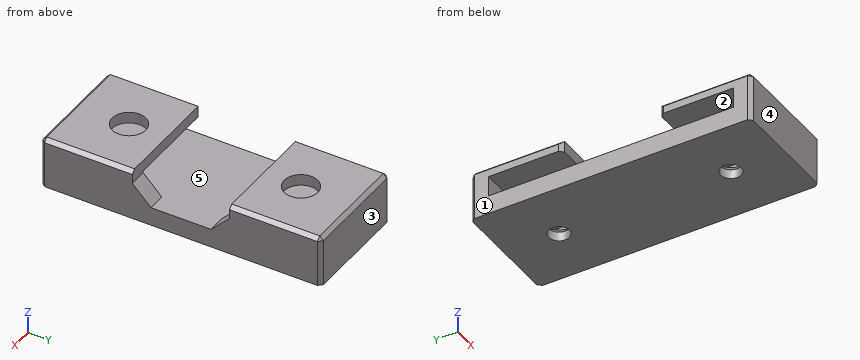
from build123d import *

# Parameters (mm, degrees)
SKETCH001_W     = 30
SKETCH001_H     = 75
SKETCH001_R     = 2.75
PAD_DEPTH       = 5
PAD001_DEPTH    = 5.5
SKETCH003_W     = 30
SKETCH003_H     = 24.5
PAD002_DEPTH    = 3
CHAMFER_SIZE    = 2.5
SKETCH004_R     = 4.5
POCKET_DEPTH    = 3
CHAMFER001_SIZE = 5
CHAMFER002_SIZE = 1


with BuildPart() as part:
    # Sketch001 → Pad (new body)
    with BuildSketch(Plane.XY):
        Rectangle(SKETCH001_W, SKETCH001_H)
        with Locations((0, 23)):
            Circle(SKETCH001_R, mode=Mode.SUBTRACT)
        with Locations((0, -23)):
            Circle(SKETCH001_R, mode=Mode.SUBTRACT)
    extrude(amount=PAD_DEPTH)

    # Sketch002 (on Face8 of Pad) → Pad001 (join)
    with BuildSketch(Plane.XY.offset(5)):
        Polygon((-15, 37.5), (15, 37.5), (15, 13), (10.25, 13), (10.25, 32.75), (-15, 32.75), align=None)
        Polygon((-15, -37.5), (15, -37.5), (15, -13), (10.25, -13), (10.25, -32.75), (-15, -32.75), align=None)
    extrude(amount=PAD001_DEPTH)

    # Sketch003 (on Face10 of Pad001) → Pad002 (join)
    with BuildSketch(Plane.XY.offset(10.5)):
        with Locations((0, 25.25)):
            Rectangle(SKETCH003_W, SKETCH003_H)
        with Locations((0, -25.25)):
            Rectangle(SKETCH003_W, SKETCH003_H)
    extrude(amount=PAD002_DEPTH)

    # Chamfer
    chamfer_edges = [part.edges().sort_by_distance(p)[0] for p in [
        (-2.75, -23, 5),
        (-2.75, 23, 5),
    ]]
    chamfer(chamfer_edges, length=CHAMFER_SIZE)

    # Sketch004 (on Face18 of Chamfer) → Pocket (cut)
    with BuildSketch(Plane.XY.offset(13.5)):
        with Locations((0, 23)):
            Circle(SKETCH004_R)
        with Locations((0, -23)):
            Circle(SKETCH004_R)
    extrude(amount=-POCKET_DEPTH, mode=Mode.SUBTRACT)

    # Chamfer001
    chamfer001_edges = [part.edges().sort_by_distance(p)[0] for p in [
        (12.625, 13, 5),
        (12.625, -13, 5),
    ]]
    chamfer(chamfer001_edges, length=CHAMFER001_SIZE)

    # Chamfer002
    chamfer002_edges = [part.edges().sort_by_distance(p)[0] for p in [
        (15, 25.25, 13.5),
        (0, 37.5, 13.5),
        (15, -25.25, 13.5),
        (0, -37.5, 13.5),
        (-15, 25.25, 13.5),
        (-15, -25.25, 13.5),
        (-15, 13, 12),
        (-15, -13, 12),
        (-15, -37.5, 6.75),
        (-15, 37.5, 6.75),
        (15, -37.5, 6.75),
        (15, 37.5, 6.75),
    ]]
    chamfer(chamfer002_edges, length=CHAMFER002_SIZE)


solid = part.part
Design review of the part built by this model. Coordinates are the model's own, in mm. Face numbers are marked on the shaded views. A direction names the side the tool comes from. Coordinates: 2 decimals unless noted, no trailing zeros. Loops run counter-clockwise (first coordinate to the right, second up) from the corner with the lowest first, then second, coordinate; pieces in that order, holes last. Notation, with made-up numbers: (34, 15.25) -> (74, 15.25) arc R5 ccw to (74, 24.25) -> close; hole circle Ø11 at (16.5, 35.25). An arc over 180 degrees is marked (long way). Use a Markdown table: item, result. Add a question column.
Item 1: The part is to be moulded in two halves that separate along Y. For the marked faces 1, 2 and 3, say which applies: +Y half, -Y half, draft (parallel to the pull), parting line (faces both ways), or undercut.
Item 2: We need section C-C, the plane y = 23. Write out the cut boundary in (x, z).
Item 3: Clearance check with flat-ended pins moving along their axes: P1, Ø1.6, axis at y = -20.5, z = 6.5, coming from the -X side; P2, Ø7, axis at x = 0, y = -23, coming from the -Z side; P3, Ø15, axis at x = 0.5, y = -3.5, coming from the +Z side; P4, Ø5, axis at y = 5, z = 8.5, coming from the +X side. State where each tip first meets the part, or that it passes through.
Item 4: We need section A-A, the plane z = 11.5. Write out the cut boundary in (x, y).
Item 5: Machinability: for the marked faces 4 and 5, which of the approach directions +Z, -Z, +X, -X, +Y, -Y give a long, thin tool a straight path to every point of the face, cutting with its end or side? Answer none if there is none.
Item 6: We need section D-D, the plane z = 3.75. Write out the cut boundary in (x, y).
Item 7: We need section B-B, the plane x = 0. Count the separate pieces of the cut face and the enclosed holes in it, and give its area (3 significant figures).
Item 8: Wall thickness on L1, parallel to Z at x = -5, y = 21; L2, parallel to Y at x = 0, z = 12.85; L3, parallel to Y at x = 2.5, z = 9.25: over which ranges is each line inside the solid? List them lowest first. Write a range as from..to.
Numbers:
| question | item | result |
|---|---|---|
| 1 | face 1 | draft |
| 1 | face 2 | undercut |
| 1 | face 3 | +Y half |
| 2 | outline | (-15, 0) -> (-2.75, 0) -> (-2.75, 2.5) -> (-5.25, 5) -> (-15, 5) -> close; (-15, 10.5) -> (-4.5, 10.5) -> (-4.5, 13.5) -> (-14, 13.5) -> (-15, 12.5) -> close; (2.75, 0) -> (15, 0) -> (15, 12.5) -> (14, 13.5) -> (4.5, 13.5) -> (4.5, 10.5) -> (10.25, 10.5) -> (10.25, 5) -> (5.25, 5) -> (2.75, 2.5) -> close |
| 3 | P1 | stops at x = 10.25 |
| 3 | P2 | stops at z = 0 |
| 3 | P3 | stops at z = 5 |
| 3 | P4 | passes through |
| 4 | outline | (-15, -36.5) -> (-14, -37.5) -> (14, -37.5) -> (15, -36.5) -> (15, -13) -> (-14, -13) -> (-15, -14) -> close; (-15, 14) -> (-14, 13) -> (15, 13) -> (15, 36.5) -> (14, 37.5) -> (-14, 37.5) -> (-15, 36.5) -> close; hole circle Ø9 at (0, -23); hole circle Ø9 at (0, 23) |
| 5 | face 4 | +Z, -Z, +X, -X, -Y |
| 5 | face 5 | -X |
| 6 | outline | (-15, -36.5) -> (-14, -37.5) -> (14, -37.5) -> (15, -36.5) -> (15, 36.5) -> (14, 37.5) -> (-14, 37.5) -> (-15, 36.5) -> close; hole circle Ø8 at (0, -23); hole circle Ø8 at (0, 23) |
| 7 | separate pieces | 5 |
| 7 | enclosed holes | 0 |
| 7 | area | 452 mm^2 |
| 8 | L1 | z = 0..5, 10.5..13.5 |
| 8 | L2 | y = -37.15..-27.5, -18.5..-13, 13..18.5, 27.5..37.15 |
| 8 | L3 | y = -37.5..-32.75, 32.75..37.5 |
